Autodesk Inventor part; units mm, degrees
ref_plane "YZ Plane" through (0, 0, 0) normal (1, 0, 0) x (0, 1, 0)
ref_plane "XZ Plane" through (0, 0, 0) normal (0, 1, 0) x (-1, 0, 0)
ref_plane "XY Plane" through (0, 0, 0) normal (0, 0, 1) x (1, 0, 0)
sketch "Sketch1" plane through (0, 0, 0) normal (0, 0, 1) x (1, 0, 0)
  line L0 (0, 0) -> (38.1, 0)
  line L1 (38.1, 0) -> (38.1, 38.1)
  line L2 (38.1, 38.1) -> (0, 38.1)
  line L3 (0, 38.1) -> (0, 0)
  dimension "d0" = 38.1
  dimension "d1" = 38.1
extrude "Extrusion1" add sketch "Sketch1" along normal blind 127
sketch "Sketch2" plane through (0, 0, 127) normal (0, 0, 1) x (1, 0, 0)
  line L0 (-0.4591, 31.2765) -> (45.936, 31.2765) construction
  line L1 (45.936, 31.2765) -> (45.936, -1.3483) construction
  line L2 (45.936, -1.3483) -> (-0.4591, -1.3483) construction
  line L3 (-0.4591, -1.3483) -> (-0.4591, 31.2765) construction
  spline S0 degree 2 poles (18.4777, 5.5554) (17.7367, 5.3742) (16.1229, 5.1766) (15.3161, 5.1766) knots 0 0 0 1 2 2 2
  spline S1 degree 2 poles (15.3161, 5.1766) (13.0272, 5.1766) (10.1784, 7.729) (10.0467, 10.1002) knots 0 0 0 1 2 2 2
  spline S2 degree 2 poles (10.0467, 10.1002) (9.8656, 10.1002) (9.5527, 10.1002) (9.421, 10.1002) knots 0 0 0 1 2 2 2
  spline S3 degree 2 poles (9.421, 10.1002) (7.3626, 10.1002) (4.0528, 11.4999) (2.8672, 12.8666) knots 0 0 0 1 2 2 2
  spline S4 degree 2 poles (2.8672, 12.8666) (1.698, 14.2169) (0.4466, 18.1689) (0.4466, 20.6719) knots 0 0 0 1 2 2 2
  spline S5 degree 2 poles (0.4466, 20.6719) (0.4466, 23.2407) (1.7145, 27.1269) (2.8837, 28.5101) knots 0 0 0 1 2 2 2
  spline S6 degree 2 poles (2.8837, 28.5101) (4.0693, 29.8768) (7.3791, 31.2765) (9.421, 31.2765) knots 0 0 0 1 2 2 2
  spline S7 degree 2 poles (9.421, 31.2765) (11.4958, 31.2765) (14.8221, 29.8274) (15.9747, 28.5101) knots 0 0 0 1 2 2 2
  spline S8 degree 2 poles (15.9747, 28.5101) (17.1274, 27.1763) (18.4118, 23.2078) (18.4118, 20.6719) knots 0 0 0 1 2 2 2
  spline S9 degree 2 poles (18.4118, 20.6719) (18.4118, 16.7198) (15.3325, 11.5822) (12.6485, 10.6765) knots 0 0 0 1 2 2 2
  spline S10 degree 2 poles (12.6485, 10.6765) (12.7143, 9.9191) (13.1095, 8.7005) (13.4224, 8.3547) knots 0 0 0 1 2 2 2
  spline S11 degree 2 poles (13.4224, 8.3547) (13.8011, 7.9266) (14.8385, 7.5314) (15.7607, 7.5314) knots 0 0 0 1 2 2 2
  spline S12 degree 2 poles (15.7607, 7.5314) (16.3041, 7.5314) (17.7861, 7.8772) (18.1154, 8.0089) knots 0 0 0 1 2 2 2
  line L4 (18.1154, 8.0089) -> (18.4777, 8.0089)
  line L5 (18.4777, 8.0089) -> (18.4777, 5.5554)
  spline S13 degree 2 poles (15.596, 20.6719) (15.596, 22.6973) (14.7233, 25.8095) (13.9329, 26.8304) knots 0 0 0 1 2 2 2
  spline S14 degree 2 poles (13.9329, 26.8304) (13.126, 27.8843) (10.8536, 28.9382) (9.4374, 28.9382) knots 0 0 0 1 2 2 2
  spline S15 degree 2 poles (9.4374, 28.9382) (7.9719, 28.9382) (5.7653, 27.9173) (4.9255, 26.8304) knots 0 0 0 1 2 2 2
  spline S16 degree 2 poles (4.9255, 26.8304) (4.1187, 25.793) (3.2624, 22.6479) (3.2624, 20.6719) knots 0 0 0 1 2 2 2
  spline S17 degree 2 poles (3.2624, 20.6719) (3.2624, 16.6704) (6.6216, 12.4056) (9.4374, 12.4056) knots 0 0 0 1 2 2 2
  spline S18 degree 2 poles (9.4374, 12.4056) (12.2532, 12.4056) (15.596, 16.6704) (15.596, 20.6719) knots 0 0 0 1 2 2 2
  line L6 (37.1016, 10.5283) -> (33.5942, 10.5283)
  line L7 (33.5942, 10.5283) -> (27.1721, 18.6135)
  line L8 (27.1721, 18.6135) -> (24.0764, 18.6135)
  line L9 (24.0764, 18.6135) -> (24.0764, 10.5283)
  line L10 (24.0764, 10.5283) -> (21.3758, 10.5283)
  line L11 (21.3758, 10.5283) -> (21.3758, 30.8483)
  line L12 (21.3758, 30.8483) -> (26.6123, 30.8483)
  spline S19 degree 2 poles (26.6123, 30.8483) (28.3578, 30.8483) (30.7125, 30.4696) (31.7828, 29.778) knots 0 0 0 1 2 2 2
  spline S20 degree 2 poles (31.7828, 29.778) (32.8532, 29.0864) (34.0882, 26.9292) (34.0882, 25.332) knots 0 0 0 1 2 2 2
  spline S21 degree 2 poles (34.0882, 25.332) (34.0882, 23.109) (31.8158, 20.0955) (29.8727, 19.371) knots 0 0 0 1 2 2 2
  line L13 (29.8727, 19.371) -> (37.1016, 10.5283)
  spline S22 degree 2 poles (31.2724, 25.1179) (31.2724, 26.0071) (30.6466, 27.3739) (29.988, 27.8185) knots 0 0 0 1 2 2 2
  spline S23 degree 2 poles (29.988, 27.8185) (29.4116, 28.1972) (27.8802, 28.5101) (26.7605, 28.5101) knots 0 0 0 1 2 2 2
  line L14 (26.7605, 28.5101) -> (24.0764, 28.5101)
  line L15 (24.0764, 28.5101) -> (24.0764, 20.8695)
  line L16 (24.0764, 20.8695) -> (26.4476, 20.8695)
  spline S24 degree 2 poles (26.4476, 20.8695) (27.6168, 20.8695) (29.4775, 21.2811) (30.1197, 21.9233) knots 0 0 0 1 2 2 2
  spline S25 degree 2 poles (30.1197, 21.9233) (30.7125, 22.4832) (31.2724, 24.064) (31.2724, 25.1179) knots 0 0 0 1 2 2 2
  point P0 (0, 0)
extrude "Extrusion2" cut sketch "Sketch2" against normal blind 2.54
properties part number "Container 2 2 5 QR color 5"
Verification items for the finished model (mm, model axes). A direction names the side the tool comes from. Coordinates: 2 decimals unless noted, no trailing zeros. Answer as a JSON object with one key per item and string values. Group by question number.
(1) Material ranges on line 1 (Z direction, x = 34, y = 13), recorded low to high.
(2) Release check for a two-part mould opening along X. For faces 3 (the face through (0, 19, 63)), 4 (the face through (28, 25, 127)), 5 (the face through (33.44, 15.01, 125.75)), 6 (the face through (23, 10.528, 126)) record: +X half, -X half, draft (parallel to the pull), parting line (faces both ways), or undercut.
(3) Tool access check on faces 1 (the face through (29, 21, 124.46)), 2 (the face through (19, 19, 0)). Record the directions out of +Z, -Z, +X, -X, +Y, -Y that give a thin tool (end or side, any length) a straight path to the whole face; none if there is none.
(4) Gauge pin test, flat end, axial feed: pin 1 (2 mm diameter, centred on y = 16, z = 125, fed in from -X). Record the tip position at first contact, or that the pin passes through.
Reply:
{
 "1": {"line 1": "0 to 124.46"},
 "2": {"face 3": "-X half", "face 4": "draft", "face 5": "undercut", "face 6": "undercut"},
 "3": {"face 1": "+Z", "face 2": "-Z, +X, -X, +Y, -Y"},
 "4": {"pin 1": "x = 0"}
}
